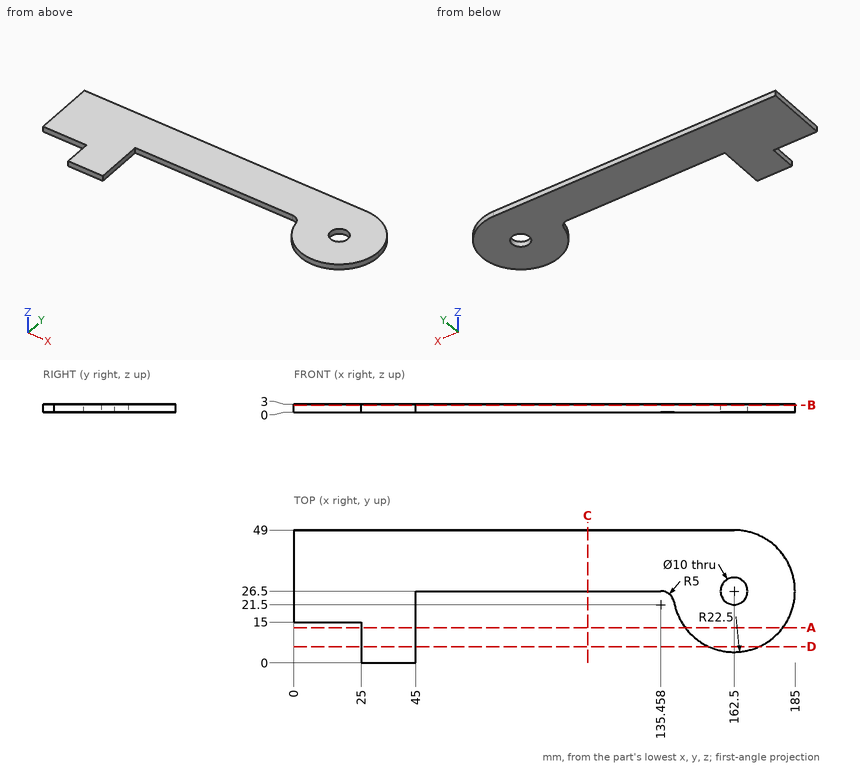
Here's the drawing with two shaded views (mm, measured from the low corner). I have some questions. Give positions to 0.01 mm unless a question says otherwise; leave off trailing zeros. Write each loop counter-clockwise with the first axis right and the second up, starting at its lowest first coordinate (ties: lowest second). Pieces come first, ordered by that corner, then holes. Notation, with made-up numbers: (80, 55.5) -> (116, 55.5) arc R23 ccw to (116, 72.5) -> close; hole circle Ø8 at (59, -16.75). An arc over 180 degrees is marked (long way). Answer as a JSON object with one key per item and string values. Group by question number.
Item 1: Suppose I cut it at A-A (y = 13). Please give me the cut outline in (x, z), plus the area to 3 significant figures.
Item 2: Please list where these lines run through material, in increasing order: line 1 (Y direction, x = 162, z = 1.85) (1 decimal); line 2 (X direction, y = 23, z = 2.85) (1 decimal); line 3 (X direction, y = 24, z = 0.25). Write a range as [from, to].
Item 3: Suppose I cut it at B-B (z = 2.55). Please give me the cut outline in (x, y) (1 decimal), plus the area to 3 significant figures.
Item 4: I'm going to push flat-ended pins straight in: P1, Ø1.5, axis at y = 9.5, z = 1, coming from the +X side; P2, Ø0.9, axis at y = 10, z = 1.5, coming from the -X side; P3, Ø1, axis at x = 147.5, z = 0.5, coming from the -Y side (1 decimal). Where does each tip first touch, or does it pass through?
Item 5: Suppose I cut it at C-C (x = 108.5). Please give me the cut outline in (y, z).
Item 6: Suppose I cut it at D-D (y = 6). Please give me the cut outline in (x, z).
Findings:
{
 "1": {"outline": "(25, 0) -> (45, 0) -> (45, 3) -> (25, 3) -> close; (144.5, 0) -> (180.5, 0) -> (180.5, 3) -> (144.5, 3) -> close", "area": "168 mm²"},
 "2": {"line 1": "y = [4, 21.5], [31.5, 49]", "line 2": "x = [0, 45], [140.2, 158.9], [166.1, 184.7]", "line 3": "x = [0, 45], [139.79, 158.17], [166.83, 184.86]"},
 "3": {"outline": "(0, 15) -> (25, 15) -> (25, 0) -> (45, 0) -> (45, 26.5) -> (135.5, 26.5) arc R5 cw to (140.4, 22.4) arc R22.5 ccw (long way) to (162.5, 49) -> (0, 49) -> close; hole circle Ø10 at (162.5, 26.5)", "area": "5,590 mm²"},
 "4": {"P1": "stops at x = 178.06", "P2": "stops at x = 25", "P3": "stops at y = 9.3"},
 "5": {"outline": "(26.5, 0) -> (49, 0) -> (49, 3) -> (26.5, 3) -> close"},
 "6": {"outline": "(25, 0) -> (45, 0) -> (45, 3) -> (25, 3) -> close; (153.23, 0) -> (171.77, 0) -> (171.77, 3) -> (153.23, 3) -> close"}
}
